Source: CAD feature listing. Evaluate the final solid. Frame: model axes, mm. A direction names the side the tool comes from. Give positions to 0.01 mm unless a question says otherwise; leave off trailing zeros. Order: outer loops, then holes, each group sorted by start corner. A loop starts at its lowest first (then second) coordinate and runs counter-clockwise, first axis right, second up. Notation, with made-up numbers: (-11.75, 16.25) -> (37.25, 16.25) arc R22 ccw to (37.25, 29.25) -> close; hole circle Ø2 at (-16, 10). An arc over 180 degrees is marked (long way). Answer in a Markdown table with one row per item.
```python
from build123d import *

# Parameters (mm, degrees)
SKIZZE1_R                       = 50
AUFSATZ_LINEAR_AUSTRAGEN1_DEPTH = 10
SKIZZE2_R                       = 1.7
SCHNITT_LINEAR_AUSTRAGEN1_DEPTH = 10
SKIZZE3_R                       = 3.25
SCHNITT_LINEAR_AUSTRAGEN2_DEPTH = 4.5
SKIZZE7_R                       = 9
SCHNITT_LINEAR_AUSTRAGEN5_DEPTH = 11
SKIZZE4_W                       = 20.4
SKIZZE4_H                       = 2.6
SCHNITT_LINEAR_AUSTRAGEN3_DEPTH = 10
AUFSATZ_LINEAR_START            = -10
SKIZZE5_R                       = 4
AUFSATZ_LINEAR_AUSTRAGEN2_DEPTH = 13
SKIZZE6_R                       = 2
SCHNITT_LINEAR_AUSTRAGEN4_DEPTH = 6


with BuildPart() as part:
    # Skizze1 → Aufsatz-Linear austragen1 (new body)
    with BuildSketch(Plane(origin=(0, 0, 0), x_dir=(1, 0, 0), z_dir=(0, 1, 0))):
        Circle(SKIZZE1_R)
    extrude(amount=AUFSATZ_LINEAR_AUSTRAGEN1_DEPTH)

    # Skizze2 → Schnitt-Linear austragen1 (cut)
    with BuildSketch(Plane(origin=(0, 10, 0), x_dir=(1, 0, 0), z_dir=(0, 1, 0))):
        with Locations((-25, 25)):
            Circle(SKIZZE2_R)
        with Locations((25, 25)):
            Circle(SKIZZE2_R)
        with Locations((25, -25)):
            Circle(SKIZZE2_R)
        with Locations((-25, -25)):
            Circle(SKIZZE2_R)
    extrude(amount=-SCHNITT_LINEAR_AUSTRAGEN1_DEPTH, mode=Mode.SUBTRACT)

    # Skizze3 → Schnitt-Linear austragen2 (cut)
    with BuildSketch(Plane(origin=(0, 10, 0), x_dir=(1, 0, 0), z_dir=(0, 1, 0))):
        with Locations((-25, 25)):
            Circle(SKIZZE3_R)
        with Locations((25, 25)):
            Circle(SKIZZE3_R)
        with Locations((25, -25)):
            Circle(SKIZZE3_R)
        with Locations((-25, -25)):
            Circle(SKIZZE3_R)
    extrude(amount=-SCHNITT_LINEAR_AUSTRAGEN2_DEPTH, mode=Mode.SUBTRACT)

    # Skizze7 → Schnitt-Linear austragen5 (cut, through all)
    with BuildSketch(Plane.XZ):
        Circle(SKIZZE7_R)
    extrude(amount=-SCHNITT_LINEAR_AUSTRAGEN5_DEPTH, mode=Mode.SUBTRACT)

    # Skizze4 → Schnitt-Linear austragen3 (cut)
    with BuildSketch(Plane(origin=(0, 10, 0), x_dir=(1, 0, 0), z_dir=(0, 1, 0))):
        with Locations((0, -6.2)):
            Rectangle(SKIZZE4_W, SKIZZE4_H)
    extrude(amount=-SCHNITT_LINEAR_AUSTRAGEN3_DEPTH, mode=Mode.SUBTRACT)

    # Skizze5 → Aufsatz-Linear austragen2 (add)
    with BuildSketch(Plane(origin=(0, 10, 0), x_dir=(1, 0, 0), z_dir=(0, 1, 0)).offset(AUFSATZ_LINEAR_START)):
        with Locations((-7.75, 5.215)):
            Circle(SKIZZE5_R)
        with BuildLine():
            ThreePointArc((-6.220782003, 6.503988874), (-9.409308992, 6.331554373), (-8.368075659, 3.312900507))
            ThreePointArc((-8.368075659, 3.312900507), (-7.466890464, 5.02449468), (-6.220782003, 6.503988874))
        make_face(mode=Mode.SUBTRACT)
        with Locations((7.75, 5.215)):
            Circle(SKIZZE5_R)
        with BuildLine():
            ThreePointArc((8.368075659, 3.312900507), (9.409308992, 6.331554373), (6.220782003, 6.503988874))
            ThreePointArc((6.220782003, 6.503988874), (7.466890464, 5.02449468), (8.368075659, 3.312900507))
        make_face(mode=Mode.SUBTRACT)
    extrude(amount=AUFSATZ_LINEAR_AUSTRAGEN2_DEPTH)

    # Skizze6 → Schnitt-Linear austragen4 (cut)
    with BuildSketch(Plane(origin=(0, 12.999999992, 0), x_dir=(1, 0, 0), z_dir=(0, 1, 0))):
        with Locations((-7.75, 5.215)):
            Circle(SKIZZE6_R)
        with Locations((7.75, 5.215)):
            Circle(SKIZZE6_R)
    extrude(amount=-SCHNITT_LINEAR_AUSTRAGEN4_DEPTH, mode=Mode.SUBTRACT)


solid = part.part
```
(1) First-contact query: pin 1 Ø4.5 at (x, z) = (-25, 25) entering from -Y; pin 2 Ø3 at (y, z) = (2, 6.5) entering from -X; pin 3 Ø2 at (x, y) = (-4, 9.5) entering from +Z; pin 4 Ø3 at (x, z) = (36, 1) entering from +Y. Flat tips, straight axial feed; report the tip coordinate or a pass-through.
A:
| item | result |
|---|---|
| pin 1 | stops at y = 0 |
| pin 2 | stops at x = -49.75 |
| pin 3 | stops at z = 49.91 |
| pin 4 | stops at y = 10 |
(2) Section query C-C (z = 37.5). Return the cut outline in (x, y), plus the area to 3 significant figures.
A:
| item | result |
|---|---|
| outline | (-33.07, 0) -> (33.07, 0) -> (33.07, 10) -> (-33.07, 10) -> close |
| area | 661 mm^2 |
(3) Section query B-B (y = 3.5). Return the cut outline in (x, z) (3 decimals), plus the area to 3 significant figures.
A:
| item | result |
|---|---|
| outline | circle Ø100 at (0, 0); hole circle Ø3.4 at (-25, -25); hole circle Ø3.4 at (-25, 25); hole (-10.2, 4.9) -> (-7.549, 4.9) arc R9 ccw to (-8.893, -1.382) arc R4 cw to (-4.63, -7.718) arc R9 ccw to (4.63, -7.718) arc R4 cw to (8.893, -1.382) arc R9 ccw to (7.549, 4.9) -> (10.2, 4.9) -> (10.2, 7.5) -> (4.975, 7.5) arc R9 ccw to (-4.975, 7.5) -> (-10.2, 7.5) -> close; hole circle Ø3.4 at (25, -25); hole circle Ø3.4 at (25, 25) |
| area | 7,580 mm^2 |
(4) Section query A-A (z = -25). Return the cut outline in (x, y).
A:
| item | result |
|---|---|
| outline | (-43.3, 0) -> (-26.7, 0) -> (-26.7, 5.5) -> (-28.25, 5.5) -> (-28.25, 10) -> (-43.3, 10) -> close; (-23.3, 0) -> (23.3, 0) -> (23.3, 5.5) -> (21.75, 5.5) -> (21.75, 10) -> (-21.75, 10) -> (-21.75, 5.5) -> (-23.3, 5.5) -> close; (26.7, 0) -> (43.3, 0) -> (43.3, 10) -> (28.25, 10) -> (28.25, 5.5) -> (26.7, 5.5) -> close |
(5) Section query D-D (x = 31). Return the cut outline in (y, z), plus the area to 3 significant figures.
A:
| item | result |
|---|---|
| outline | (0, -39.23) -> (10, -39.23) -> (10, 39.23) -> (0, 39.23) -> close |
| area | 785 mm^2 |
(6) Ray query, probe 1 along X at (y, z) = (5.5, 0); probe 2 along X at (y, z) = (3.8, -25); probe 3 along Z at (x, y) = (22.5, 6.75). Return the intervals inside material, ascending.
A:
| item | result |
|---|---|
| probe 1 | x = -50 to -9, 9 to 50 |
| probe 2 | x = -43.3 to -26.7, -23.3 to 23.3, 26.7 to 43.3 |
| probe 3 | z = -44.65 to -27.08, -22.92 to 22.92, 27.08 to 44.65 |
(7) Access query for faces 1 (the flat face through (-8, 7, -5)), 2 (the flat face through (-8, 5, 7.5)). Directions: +Z, -Z, +X, -X, +Y, -Y. A direction counts if a zero-diameter tool reaches every point of the face in a straight line with its end or side. Return the directions, or none.
A:
| item | result |
|---|---|
| face 1 | +Y |
| face 2 | +Y, -Y |
(8) Pull-direction query (X, two-part tool) for faces 3 (the flat face through (-1, 0, 10)), 4 (the cylindrical face through (47.69, 4.93, -15.02)), 5 (the cylindrical face through (-27.579, 7.781, 26.978)); classes: +X half, -X half, draft (parallel to the pull), parting line (faces both ways), or undercut.
A:
| item | result |
|---|---|
| face 3 | draft |
| face 4 | parting line |
| face 5 | undercut |
